Geometry check sheet. Reference: the model listing, model coordinates, mm. A direction names the side the tool comes from. Round coordinates to 2 decimals unless told otherwise and drop trailing zeros. Loops run counter-clockwise (first coordinate to the right, second up) from the corner with the lowest first, then second, coordinate; pieces in that order, holes last. Notation, with made-up numbers: M 43,18 L 77,18 A21 ccw 77,39 Z; hole C 3,63.25 d8. An arc over 180 degrees is marked long. Write item = value, one per line.
from build123d import *

# Parameters (mm, degrees)
F0_R      = 60
F1_DEPTH  = 70
F2_R      = 60
F3_DEPTH  = 70
F3_TAPER  = 7
F5_R      = 54.9341030365
F6_DEPTH  = 25.4
F7_R      = 47.9617586767
F8_DEPTH  = 205.994
F4_R      = 51.4050807368
F12_DEPTH = 50
F13_R     = 51.4050807368
F14_DEPTH = 25.4
F14_TAPER = -7
F15_R     = 53.9269190887
F16_DEPTH = 70
F16_TAPER = -7
F11_R     = 60
F17_DEPTH = 25.4
F17_TAPER = -3


with BuildPart() as f1:
    # F0 (on Front) → F1 (new body)
    with BuildSketch(Plane.XZ):
        Circle(F0_R)
    extrude(amount=-F1_DEPTH)

    # F2 (on face) → F3 (join)
    with BuildSketch(Plane.XZ):
        Circle(F2_R)
    extrude(amount=F3_DEPTH, taper=F3_TAPER)

    # F5 (on face) → F6 (cut)
    with BuildSketch(Plane(origin=(0, 70, 0), x_dir=(-1, 0, 0), z_dir=(0, 1, 0))):
        Circle(F5_R)
    extrude(amount=-F6_DEPTH, mode=Mode.SUBTRACT)

    # F7 (on face) → F8 (cut)
    with BuildSketch(Plane.XZ.offset(70)):
        Circle(F7_R)
    extrude(amount=-F8_DEPTH, mode=Mode.SUBTRACT)

    # F4 (on face) → F12 (join)
    with BuildSketch(Plane.XZ.offset(70)):
        Circle(F4_R)
    extrude(amount=F12_DEPTH)

    # F13 (on face) → F14 (join)
    with BuildSketch(Plane.XZ.offset(120)):
        Circle(F13_R)
    extrude(amount=F14_DEPTH, taper=F14_TAPER)

    # F15 (on face) → F16 (join)
    with BuildSketch(Plane.XZ.offset(145.4)):
        Circle(F15_R)
    extrude(amount=F16_DEPTH, taper=F16_TAPER)

    # F11 (on face) → F17 (join)
    with BuildSketch(Plane(origin=(0, 70, 0), x_dir=(-1, 0, 0), z_dir=(0, 1, 0))):
        Circle(F11_R)
    extrude(amount=F17_DEPTH, taper=F17_TAPER)


solid = f1.part
(1) Sectioned sample at A-A on x = 0. Record the cut outline in (y, z).
Result set:
outline = M -215.4,-62.52 L -145.4,-53.93 L -145.4,-54.52 L -120,-51.41 L -70,-51.41 L 0,-60 L 70,-60 L 95.4,-61.33 L 95.4,61.33 L 70,60 L 0,60 L -70,51.41 L -120,51.41 L -145.4,54.52 L -145.4,53.93 L -215.4,62.52 Z; hole M -70,-47.96 L 44.6,-47.96 L 44.6,-54.93 L 70,-54.93 L 70,54.93 L 44.6,54.93 L 44.6,47.96 L -70,47.96 Z
(2) Material ranges on line 1 along Y through (x, z) = (17.5, -16); line 2 along Y through (x, z) = (31.5, 39); line 3 along Z through (x, y) = (0, 56), recorded low to high. Write a range as from..to.
Result set:
line_1 = -215.4..-70, 70..95.4
line_2 = -215.4..44.6, 70..95.4
line_3 = -60..-54.93, 54.93..60
(3) Sectioned sample at C-C on y = -153.5. Record the cut outline in (x, z), then the cut area to 3 significant figures.
Result set:
outline = C 0,0 d109.84
area = 9,480 mm2
(4) Tool access check on faces 4 (the cylindrical face through (-59.94, 34.51, 2.64)), 5 (the flat face through (1, 95.4, 1)). Record the directions out of +Z, -Z, +X, -X, +Y, -Y that give a thin tool (end or side, any length) a straight path to the whole face; none if there is none.
Result set:
face_4 = none
face_5 = +Z, -Z, +X, -X, +Y
(5) Sectioned sample at B-B on y = -60.5. Record the cut outline in (x, z).
Result set:
outline = C 0,0 d105.14; hole C 0,0 d95.92
(6) Depth check by flat-ended pin: pin 1 Ø12 at (y, z) = (-68, -34.5) entering from +X; pin 2 Ø4 at (y, z) = (39.5, -35.5) entering from -X; pin 3 Ø6 at (y, z) = (2, 42.5) entering from +X. Enter the tip coordinate at first touch or a pass-through.
Result set:
pin_1 = 43.17
pin_2 = -49.78
pin_3 = 45.16
(7) Release check for a two-part mould opening along Z. For faces 1 (the conical face through (13.12, 80.06, -59.09)), 2 (the flat face through (-1, -70, 1)), 3 (the flat face through (-1, -215.4, 1)) record: released by +Z, released by -Z, zero draft, split by the parting line, or undercut.
Result set:
face_1 = split by the parting line
face_2 = undercut
face_3 = zero draft
